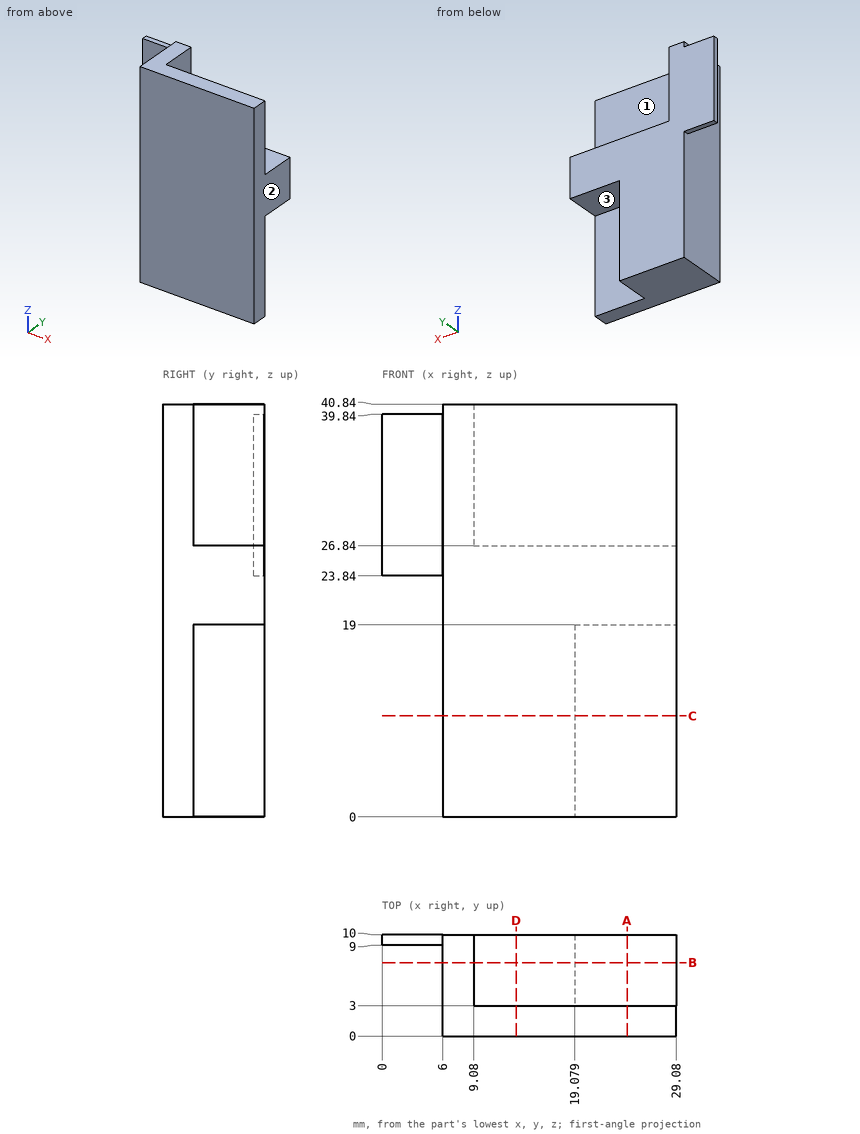
For this review, use the dimensioned drawing (mm, ordinates from the lowest corner) and the shaded views. A direction names the side the tool comes from. Round coordinates to 2 decimals unless told otherwise and drop trailing zeros. Order: outer loops, then holes, each group sorted by start corner. A loop starts at its lowest first (then second) coordinate and runs counter-clockwise, first axis right, second up. Notation, with made-up numbers: M 68.25,20.5 L 80.25,20.5 A17 cw 80.25,44.5 Z; hole C 68.5,-26.75 d9. An arc over 180 degrees is marked long. Use a Markdown table: item, result. Add a question column.
Item 1: Add section C-C, the plane z = 10. Give the boundary of the cut face in (x, y), then the cut area to 3 significant figures.
Item 2: Add section A-A, the plane x = 24.25. Give the boundary of the cut face in (y, z).
Item 3: Add section D-D, the plane x = 13.25. Give the boundary of the cut face in (y, z).
Item 4: Insertion check: pin 1 (8 mm diameter, centred on x = 23.5, z = 7.5, fed in from +Y); pin 2 (2 mm diameter, centred on x = 17.5, y = 6, fed in from +Z); pin 3 (3.5 mm diameter, centred on x = 23, y = 7.5, fed in from -Z). Each pin has a flat end and moves straight along its axis. Give the tip position at first contact, or say it passes through.
Item 5: Add section B-B, the plane y = 7.25. Give the boundary of the cut face in (x, z).
Item 6: To check wall thickness, follow line 1 along X through (y, z) = (4, 23); line 2 along Y through (x, z) = (20.5, 15); line 3 along Z through (x, y) = (13.5, 5.25). State the ranges of each line that lie inside material, in increasing order.
Item 7: Tool access review of the marked faces 1, 2 and 3: name each direction out of +Z, -Z, +X, -X, +Y, -Y from which nothing blocks a thin tool from reaching the whole face with its end or side.
Geometry results:
| question | item | result |
|---|---|---|
| 1 | outline | M 6,0 L 29.08,0 L 29.08,3 L 19.08,3 L 19.08,10 L 6,10 Z |
| 1 | area | 161 mm² |
| 2 | outline | M 0,0 L 3,0 L 3,19 L 10,19 L 10,26.84 L 3,26.84 L 3,40.84 L 0,40.84 Z |
| 3 | outline | M 0,0 L 10,0 L 10,26.84 L 3,26.84 L 3,40.84 L 0,40.84 Z |
| 4 | pin 1 | stops at y = 3 |
| 4 | pin 2 | stops at z = 26.84 |
| 4 | pin 3 | stops at z = 19 |
| 5 | outline | M 6,0 L 19.08,0 L 19.08,19 L 29.08,19 L 29.08,26.84 L 9.08,26.84 L 9.08,40.84 L 6,40.84 Z |
| 6 | line 1 | x = 6 to 29.08 |
| 6 | line 2 | y = 0 to 3 |
| 6 | line 3 | z = 0 to 26.84 |
| 7 | face 1 | +Z, +X, +Y |
| 7 | face 2 | +Z, -Z, +X, +Y, -Y |
| 7 | face 3 | -Z, +X, +Y |
